Source: CAD feature listing. Evaluate the final solid. Frame: model axes, mm. Face numbers are marked on the shaded views. A direction names the side the tool comes from. Coordinates: 2 decimals unless noted, no trailing zeros. Loops run counter-clockwise (first coordinate to the right, second up) from the corner with the lowest first, then second, coordinate; pieces in that order, holes last.
Item 1: Section query C-C, the plane z = 19.5. Return the cut outline in (x, y), then the cut area to 3 significant figures.
Item 2: Reachability of the marked faces 1 and 2 from +Z, -Z, +X, -X, +Y, -Y: full face, straight path, thin tool, end or side. Return the list, or none.
Item 3: Pin query (flat end, axial travel): pin 1 Ø19 at (x, y) = (13, 36) entering from -Z. Return the tip coordinate at first contact, or that it passes through.
Item 4: Line query: probe 1 along X at (y, z) = (7, 20); probe 2 along Z at (x, y) = (132, -134.5). Output: solid intervals per line, ascending.
Item 5: Section query B-B, the plane y = -105. Return the cut outline in (x, z), then the cut area to 3 significant figures.
Item 6: Section query A-A, the plane x = -97.5. Return the cut outline in (y, z).
Item 7: Section query D-D, the plane y = -137. Return the cut outline in (x, z), then the cut area to 3 significant figures.
Item 8: Pull-direction query (X, two-part tool) for the marked faces 3 and 4; classes: +X half, -X half, draft (parallel to the pull), parting line (faces both ways), or undercut.
```python
from build123d import *

# Parameters (mm, degrees)
F0_W     = 317.5
F0_H     = 317.5
F0_W_2   = 266.7
F0_H_2   = 266.7
F1_DEPTH = 25.4
F2_W     = 63.5
F2_H     = 317.5
F3_DEPTH = 1


with BuildPart() as f1:
    # F0 (on Top) → F1 (new body)
    with BuildSketch(Plane.XY):
        Rectangle(F0_W, F0_H)
        Rectangle(F0_W_2, F0_H_2, mode=Mode.SUBTRACT)
    extrude(amount=F1_DEPTH)

    # F2 (on face) → F3 (join)
    with BuildSketch(Plane.XY.offset(25.4)):
        Rectangle(F2_W, F2_H)
    extrude(amount=F3_DEPTH)


solid = f1.part
```
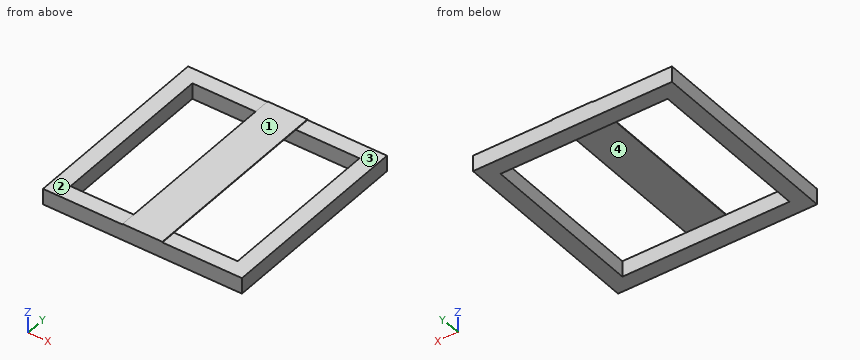
Verdict:
1. outline: (-158.75, -158.75) - (158.75, -158.75) - (158.75, 158.75) - (-158.75, 158.75) - close; hole (-133.35, -133.35) - (133.35, -133.35) - (133.35, 133.35) - (-133.35, 133.35) - close
1. area: 29,700 mm2
2. face 1: +Z, +X, -X, +Y, -Y
2. face 2: +Z, -X, +Y, -Y
3. pin 1: stops at z = 25.4
4. probe 1: x = -158.75 to -133.35, 133.35 to 158.75
4. probe 2: z = 0 to 25.4
5. outline: (-158.75, 0) - (-133.35, 0) - (-133.35, 25.4) - (-158.75, 25.4) - close; (-31.75, 25.4) - (31.75, 25.4) - (31.75, 26.4) - (-31.75, 26.4) - close; (133.35, 0) - (158.75, 0) - (158.75, 25.4) - (133.35, 25.4) - close
5. area: 1,350 mm2
6. outline: (-158.75, 0) - (-133.35, 0) - (-133.35, 25.4) - (-158.75, 25.4) - close; (133.35, 0) - (158.75, 0) - (158.75, 25.4) - (133.35, 25.4) - close
7. outline: (-158.75, 0) - (158.75, 0) - (158.75, 25.4) - (31.75, 25.4) - (31.75, 26.4) - (-31.75, 26.4) - (-31.75, 25.4) - (-158.75, 25.4) - close
7. area: 8,130 mm2
8. face 3: draft
8. face 4: undercut
